The model under review builds one solid part; all positions refer to its coordinate system, in mm. A direction names the side the tool comes from. Coordinates: 2 decimals unless noted, no trailing zeros. Order: outer loops, then holes, each group sorted by start corner. A loop starts at its lowest first (then second) coordinate and runs counter-clockwise, first axis right, second up. Notation, with made-up numbers: (-38.75, -12.5) -> (-4.75, -12.5) arc R31 ccw to (-4.75, 25.5) -> close; hole circle Ø4 at (20, -39). An arc over 180 degrees is marked (long way). Put each result on its own line as item: value.
from build123d import *

# Parameters (mm, degrees)
SKETCH2_R           = 6.35
BOSS_EXTRUDE1_DEPTH = 9.525
BOSS_EXTRUDE2_START = 9.525
SKETCH3_R           = 12.7
SKETCH3_R_2         = 6.35
BOSS_EXTRUDE2_DEPTH = 9.525


with BuildPart() as part:
    # Sketch2 → Boss-Extrude1 (new body)
    with BuildSketch(Plane.XY):
        with BuildLine():
            Line((-3.81, 37.846), (-3.81, 76.104690394))
            ThreePointArc((-3.81, 76.104690394), (-6.781597981, 75.897627953), (-9.742832479, 75.574580484))
            ThreePointArc((-9.742832479, 75.574580484), (-28.2575, 48.943425695), (-60.57809034, 46.224830674))
            ThreePointArc((-60.57809034, 46.224830674), (-62.338474903, 43.821850106), (-64.003595229, 41.351901986))
            Line((-64.003595229, 41.351901986), (-30.870597432, 22.222556788))
            ThreePointArc((-30.870597432, 22.222556788), (-29.476040643, 17.018), (-34.680597432, 15.623443212))
            Line((-34.680597432, 15.623443212), (-67.813595229, 34.752788409))
            ThreePointArc((-67.813595229, 34.752788409), (-69.120072885, 32.075777846), (-70.320922819, 29.34974981))
            ThreePointArc((-70.320922819, 29.34974981), (-56.515, 0), (-70.320922819, -29.34974981))
            ThreePointArc((-70.320922819, -29.34974981), (-69.120072885, -32.075777846), (-67.813595229, -34.752788409))
            Line((-67.813595229, -34.752788409), (-34.680597432, -15.623443212))
            ThreePointArc((-34.680597432, -15.623443212), (-29.476040643, -17.018), (-30.870597432, -22.222556788))
            Line((-30.870597432, -22.222556788), (-64.003595229, -41.351901986))
            ThreePointArc((-64.003595229, -41.351901986), (-62.338474903, -43.821850106), (-60.57809034, -46.224830674))
            ThreePointArc((-60.57809034, -46.224830674), (-28.2575, -48.943425695), (-9.742832479, -75.574580484))
            ThreePointArc((-9.742832479, -75.574580484), (-6.781597981, -75.897627953), (-3.81, -76.104690394))
            Line((-3.81, -76.104690394), (-3.81, -37.846))
            ThreePointArc((-3.81, -37.846), (0, -34.036), (3.81, -37.846))
            Line((3.81, -37.846), (3.81, -76.104690394))
            ThreePointArc((3.81, -76.104690394), (6.781597981, -75.897627953), (9.742832479, -75.574580484))
            ThreePointArc((9.742832479, -75.574580484), (28.2575, -48.943425695), (60.57809034, -46.224830674))
            ThreePointArc((60.57809034, -46.224830674), (62.338474903, -43.821850106), (64.003595229, -41.351901986))
            Line((64.003595229, -41.351901986), (30.870597432, -22.222556788))
            ThreePointArc((30.870597432, -22.222556788), (29.476040643, -17.018), (34.680597432, -15.623443212))
            Line((34.680597432, -15.623443212), (67.813595229, -34.752788409))
            ThreePointArc((67.813595229, -34.752788409), (69.120072885, -32.075777846), (70.320922819, -29.34974981))
            ThreePointArc((70.320922819, -29.34974981), (56.515, 0), (70.320922819, 29.34974981))
            ThreePointArc((70.320922819, 29.34974981), (69.120072885, 32.075777846), (67.813595229, 34.752788409))
            Line((67.813595229, 34.752788409), (34.680597432, 15.623443212))
            ThreePointArc((34.680597432, 15.623443212), (29.476040643, 17.018), (30.870597432, 22.222556788))
            Line((30.870597432, 22.222556788), (64.003595229, 41.351901986))
            ThreePointArc((64.003595229, 41.351901986), (62.338474903, 43.821850106), (60.57809034, 46.224830674))
            ThreePointArc((60.57809034, 46.224830674), (28.2575, 48.943425695), (9.742832479, 75.574580484))
            ThreePointArc((9.742832479, 75.574580484), (6.781597981, 75.897627953), (3.81, 76.104690394))
            Line((3.81, 76.104690394), (3.81, 37.846))
            ThreePointArc((3.81, 37.846), (0, 34.036), (-3.81, 37.846))
        make_face()
        with Locations(Location((0, 0, 0), (0, 0, 180))):
            Circle(SKETCH2_R, mode=Mode.SUBTRACT)
    extrude(amount=BOSS_EXTRUDE1_DEPTH)

    # Sketch3 → Boss-Extrude2 (add)
    with BuildSketch(Plane(origin=(0, 0, 0), x_dir=(-1, 0, 0), z_dir=(0, 0, -1)).offset(BOSS_EXTRUDE2_START)):
        with Locations(Location((0, 0, 0), (0, 0, 180))):
            Circle(SKETCH3_R)
        Circle(SKETCH3_R_2, mode=Mode.SUBTRACT)
    extrude(amount=-BOSS_EXTRUDE2_DEPTH)


solid = part.part
Item 1: Mouldability with a two-part tool opening along X and no side actions: class faces 1 (the cylindrical face through (-62.36, -43.79, 4.7)), 2 (the flat face through (15, 1, 0)), 3 (the flat face through (3.81, -57, 5)) as +X half, -X half, draft (parallel to the pull), parting line (faces both ways), or undercut.
Answers below:
face 1: -X half
face 2: draft
face 3: undercut
Item 2: Consider section D-D on y = 58.5. Write out the cut boundary in (x, z) (3 decimals).
Answers below:
outline: (-17.27, 0) -> (-3.81, 0) -> (-3.81, 9.525) -> (-17.27, 9.525) -> close; (3.81, 0) -> (17.27, 0) -> (17.27, 9.525) -> (3.81, 9.525) -> close
Item 3: For faces 4 (the flat face through (-47.67, 31.92, 4.7)), 5 (the flat face through (3.81, 57, 5)), 6 (the cylindrical face through (69.103, -32.114, 4.696)), 7 (the cylindrical face through (-56.518, 0.469, 4.696)), 8 (the cylindrical face through (5.86, 11.267, -4.829)), list the 3-axis set-ups (+Z, -Z, +X, -X, +Y, -Y) from which the entire face can be reached by the end or side of a thin tool; tool diameter is ignored.
Answers below:
face 4: +Z, -Z
face 5: +Z, -Z, +Y
face 6: +Z, -Z, +X, -Y
face 7: +Z, -Z, -X
face 8: -Z
Item 4: For line 1 (Y direction, x = 0, z = -7); line 2 (Y direction, x = -38, z = 7); line 3 (Y direction, x = 0, z = 3.5), list the stretches that pass through material, from the lowest coordinate up. Write a range as from..to.
Answers below:
line 1: -12.7..-6.35, 6.35..12.7
line 2: -44.99..-26.34, -17.54..17.54, 26.34..44.99
line 3: -34.04..-6.35, 6.35..34.04
Item 5: Consider section B-B on y = 0. Write out the cut boundary in (x, z) (3 decimals), and give its area (3 significant figures).
Answers below:
outline: (-56.515, 0) -> (-12.7, 0) -> (-12.7, -9.525) -> (-6.35, -9.525) -> (-6.35, 9.525) -> (-56.515, 9.525) -> close; (6.35, -9.525) -> (12.7, -9.525) -> (12.7, 0) -> (56.515, 0) -> (56.515, 9.525) -> (6.35, 9.525) -> close
area: 1,080 mm^2
Item 6: Consider section C-C on x = 52. Write out the cut boundary in (y, z) (3 decimals), and give its area (3 significant figures).
Answers below:
outline: (-44.129, 0) -> (-34.422, 0) -> (-34.422, 9.525) -> (-44.129, 9.525) -> close; (-25.623, 0) -> (25.623, 0) -> (25.623, 9.525) -> (-25.623, 9.525) -> close; (34.422, 0) -> (44.129, 0) -> (44.129, 9.525) -> (34.422, 9.525) -> close
area: 673 mm^2
Item 7: Consider section A-A on x = 0. Write out the cut boundary in (y, z) (3 decimals).
Answers below:
outline: (-34.036, 0) -> (-12.7, 0) -> (-12.7, -9.525) -> (-6.35, -9.525) -> (-6.35, 9.525) -> (-34.036, 9.525) -> close; (6.35, -9.525) -> (12.7, -9.525) -> (12.7, 0) -> (34.036, 0) -> (34.036, 9.525) -> (6.35, 9.525) -> close
Item 8: For pin 1 Ø3 at (y, z) = (-57, 3) entering from -X; pin 2 Ø10 at (y, z) = (-19.5, 4.5) entering from +X; pin 3 Ø3 at (y, z) = (53, 6) entering from -X; pin 4 Ø6 at (y, z) = (-28, -2) entering from +X, all flat-tipped, find the tip position at first contact; note any pin that passes through.
Answers below:
pin 1: x = -19.87
pin 2: x = 65.44
pin 3: x = -24.39
pin 4: x = 70.32
